Part print with two shaded views. Sizes in mm from the minimum x, y, z corner. Give positions to 0.01 mm unless a question says otherwise; leave off trailing zeros. Answer as a JSON object with one key per item and string values.
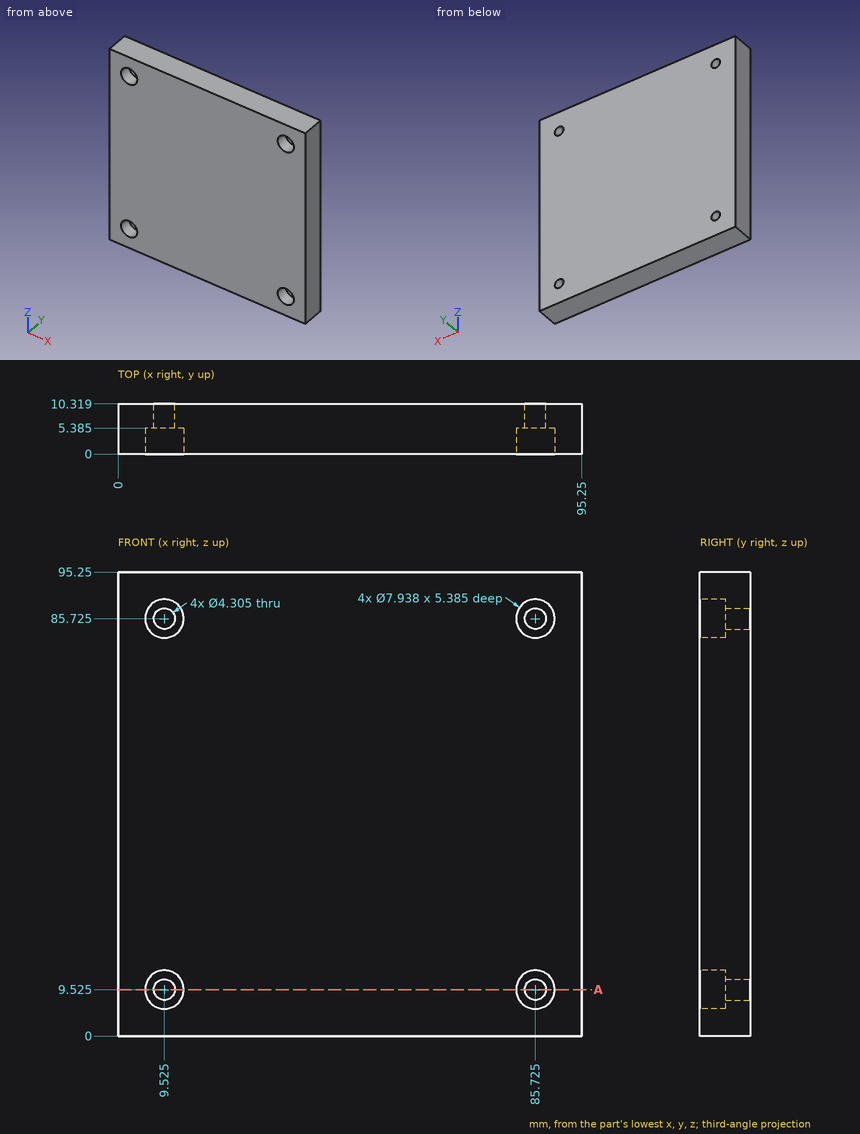
1) Slice it at A-A (z = 9.5). State how many separate pieces and enclosed holes the cut face has, then the cut area to 3 significant figures.
Model answer:
{"separate pieces": "3", "enclosed holes": "0", "area": "855 mm2"}
2) Pin check, flat tip, straight feed: pin 1 (4 mm diameter, centred on x = 10, z = 86, fed in from -Y) (1 decimal). Stop position of the tip, or through.
Model answer:
{"pin 1": "stops at y = 5.4"}
3) Wall check: probe 1 along Z at (x, y) = (9, 7.75); probe 2 along Z at (x, y) = (8.5, 3.75). Give the ranges that are in metal, low to high.
Model answer:
{"probe 1": "z = 0 to 7.44, 11.61 to 83.64, 87.81 to 95.25", "probe 2": "z = 0 to 5.69, 13.36 to 81.89, 89.56 to 95.25"}
